The drawing under review shows one solid part. Ordinate dimensions are in mm from its lowest x, y, z. A direction names the side the tool comes from. Give positions to 0.01 mm unless a question says otherwise; leave off trailing zeros. Loops run counter-clockwise (first coordinate to the right, second up) from the corner with the lowest first, then second, coordinate; pieces in that order, holes last. Notation, with made-up numbers: (61.5, 26.25) -> (96.5, 26.25) arc R13 cw to (96.5, 39.25) -> close; hole circle Ø5 at (39, 64.25). An arc over 180 degrees is marked (long way). Answer in a Markdown table with one row per item. Add a question column.
(1) Consider section A-A on x = 34. Write out the cut boundary in (y, z) (3 decimals), then the cut area to 3 significant figures.
(2) Consider section C-C on z = 18. Write out the cut boundary in (x, y), then the cut area to 3 significant figures.
(3) Consider section B-B on y = 2.25. Write out the cut boundary in (x, z), then the cut area to 3 significant figures.
(4) For line 1 (Z direction, x = 62, y = 10.7) (3 decimals); line 2 (Z direction, x = 62, y = 2.1); line 3 (Z direction, x = 34, y = 3.2), list the stretches that pass through material, from the lowest coordinate up.
(5) For the marked faces 4 and 5, list the 3-axis set-ups (+Z, -Z, +X, -X, +Y, -Y) from which the entire face can be reached by the end or side of a thin tool; tool diameter is ignored.
(6) Draft analysis for pull direction Y (two halves, no side actions). For the marked faces 1, 2 and 3, state which applies: +Y half, -Y half, draft (parallel to the pull), parting line (faces both ways), or undercut.
(7) Consider section D-D on y = 7.25. Write out the cut boundary in (x, z) (3 decimals), then the cut area to 3 significant figures.
(8) For pin 1 (1 mm diameter, centred on x = 47, y = 7.5, fed in from -Z); pin 2 (6.5 mm diameter, centred on x = 62, z = 8, fed in from -Y); pin 3 (17.5 mm diameter, centred on x = 34.5, z = 16.5, fed in from -Y), all flat-tipped, find the tip position at first contact; note any pin that passes through.
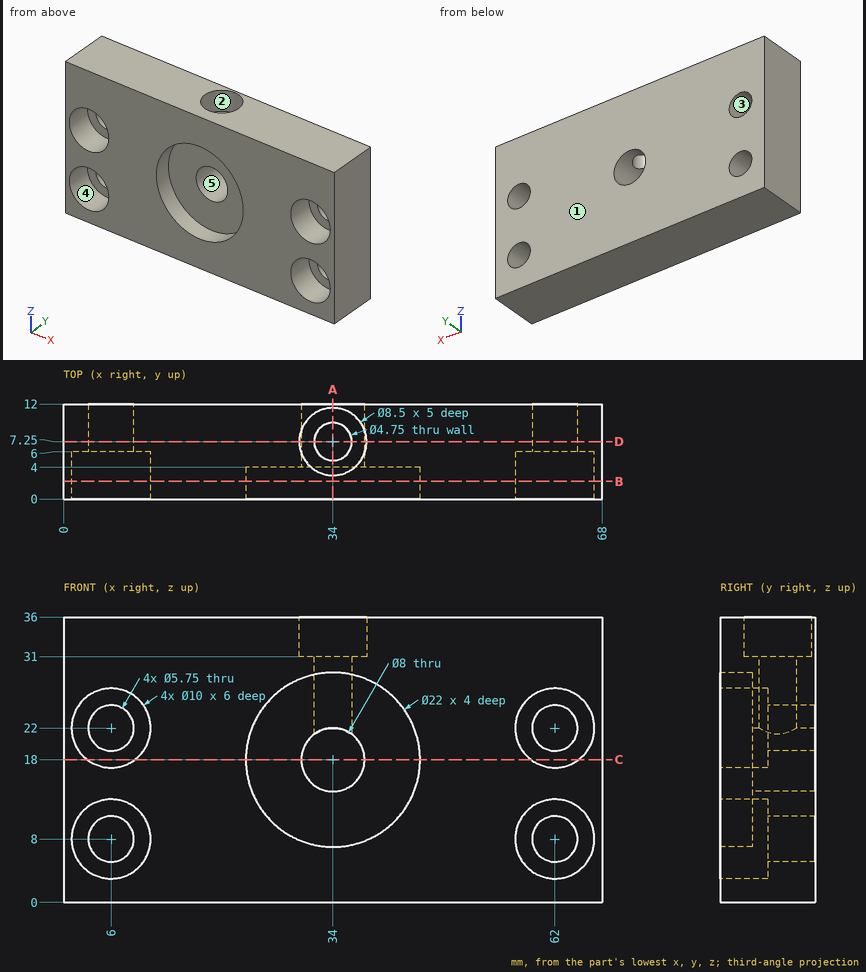
Values follow:
| question | item | result |
|---|---|---|
| 1 | outline | (0, 0) -> (12, 0) -> (12, 14) -> (4, 14) -> (4, 7) -> (0, 7) -> close; (0, 29) -> (4, 29) -> (4, 22) -> (4.875, 22) -> (4.875, 31) -> (3, 31) -> (3, 36) -> (0, 36) -> close; (9.625, 22) -> (12, 22) -> (12, 36) -> (11.5, 36) -> (11.5, 31) -> (9.625, 31) -> close |
| 1 | area | 195 mm2 |
| 2 | outline | (0, 0) -> (3, 0) -> (3, 6) -> (9, 6) -> (9, 0) -> (23, 0) -> (23, 4) -> (30, 4) -> (30, 12) -> (0, 12) -> close; (38, 4) -> (45, 4) -> (45, 0) -> (59, 0) -> (59, 6) -> (65, 6) -> (65, 0) -> (68, 0) -> (68, 12) -> (38, 12) -> close |
| 2 | area | 592 mm2 |
| 3 | outline | (0, 0) -> (68, 0) -> (68, 36) -> (0, 36) -> close; hole circle Ø10 at (6, 8); hole circle Ø10 at (6, 22); hole circle Ø22 at (34, 18); hole circle Ø10 at (62, 8); hole circle Ø10 at (62, 22) |
| 3 | area | 1,750 mm2 |
| 4 | line 1 | 0 to 5.125, 10.875 to 19.125, 24.875 to 36 |
| 4 | line 2 | 0 to 3, 13 to 17, 27 to 36 |
| 4 | line 3 | 0 to 7, 29 to 31 |
| 5 | face 4 | -Y |
| 5 | face 5 | +Y, -Y |
| 6 | face 1 | +Y half |
| 6 | face 2 | undercut |
| 6 | face 3 | draft |
| 7 | outline | (0, 0) -> (68, 0) -> (68, 36) -> (38.25, 36) -> (38.25, 31) -> (36.375, 31) -> (36.375, 21.219) arc R4 cw (long way) to (31.625, 21.219) -> (31.625, 31) -> (29.75, 31) -> (29.75, 36) -> (0, 36) -> close; hole circle Ø5.75 at (6, 8); hole circle Ø5.75 at (6, 22); hole circle Ø5.75 at (62, 8); hole circle Ø5.75 at (62, 22) |
| 7 | area | 2,210 mm2 |
| 8 | pin 1 | z = 0 |
| 8 | pin 2 | y = 6 |
| 8 | pin 3 | y = 4 |
